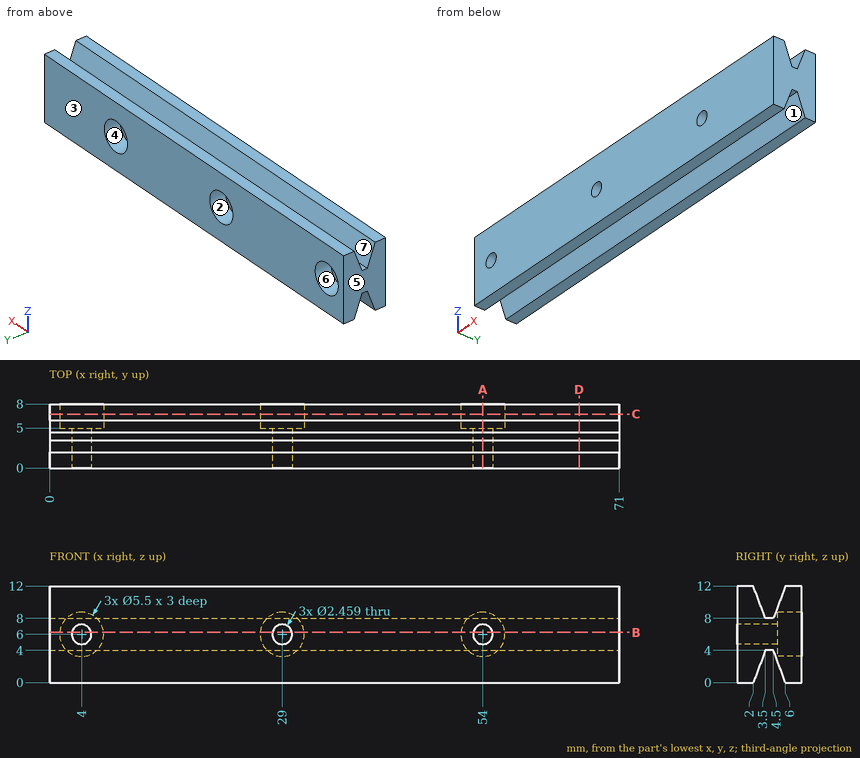
Print and shaded views of the part. All mm, measured from the part's lowest x, y and z. A direction names the side the tool comes from. Round coordinates to 2 decimals unless told otherwise and drop trailing zeros. Write each loop counter-clockwise with the first axis right and the second up, starting at its lowest first coordinate (ties: lowest second). Pieces come first, ordered by that corner, then holes. Notation, with made-up numbers: (2.25, 32) - (45.25, 32) arc R13 ccw to (45.25, 38) - close; hole circle Ø4 at (7, -9). An arc over 180 degrees is marked (long way). One line per question, with ' | ' between items.
1. Mould opens along Z. For the marked faces 4, 5, 6 and 7 say: released by +Z, released by -Z, zero draft, split by the parting line, or undercut.
Results are:
face 4: undercut | face 5: zero draft | face 6: undercut | face 7: released by +Z
2. Band-saw the part on D-D, the plane x = 66. Write the cut outline in (y, z), and give its area (3 significant figures).
Results are:
outline: (0, 0) - (2, 0) - (3.5, 4) - (4.5, 4) - (6, 0) - (8, 0) - (8, 12) - (6, 12) - (4.5, 8) - (3.5, 8) - (2, 12) - (0, 12) - close | area: 76.0 mm^2
3. Drop flat-ended pins along their axis: pin 1 Ø3 at (x, z) = (54, 6) entering from +Y; pin 2 Ø2 at (x, z) = (29, 6) entering from +Y; pin 3 Ø0.8 at (x, y) = (32.5, 4) entering from +Z. Give the stop position or say it passes through.
Results are:
pin 1: y = 5 | pin 2: through | pin 3: z = 8
4. Band-saw the part on A-A, the plane x = 54. Write the cut outline in (y, z).
Results are:
outline: (0, 0) - (2, 0) - (3.5, 4) - (4.5, 4) - (6, 0) - (8, 0) - (8, 3.25) - (5, 3.25) - (5, 4.77) - (0, 4.77) - close; (0, 7.23) - (5, 7.23) - (5, 8.75) - (8, 8.75) - (8, 12) - (6, 12) - (4.5, 8) - (3.5, 8) - (2, 12) - (0, 12) - close
5. Band-saw the part on C-C, the plane y = 6.75. Write the cut outline in (x, z).
Results are:
outline: (0, 0) - (71, 0) - (71, 12) - (0, 12) - close; hole circle Ø5.5 at (4, 6); hole circle Ø5.5 at (29, 6); hole circle Ø5.5 at (54, 6)
6. Band-saw the part on B-B, the plane z = 6.25. Write the cut outline in (x, y), and give its area (3 significant figures).
Results are:
outline: (0, 0) - (2.8, 0) - (2.8, 5) - (1.26, 5) - (1.26, 8) - (0, 8) - close; (5.2, 0) - (27.8, 0) - (27.8, 5) - (26.26, 5) - (26.26, 8) - (6.74, 8) - (6.74, 5) - (5.2, 5) - close; (30.2, 0) - (52.8, 0) - (52.8, 5) - (51.26, 5) - (51.26, 8) - (31.74, 8) - (31.74, 5) - (30.2, 5) - close; (55.2, 0) - (71, 0) - (71, 8) - (56.74, 8) - (56.74, 5) - (55.2, 5) - close | area: 483 mm^2
7. Tool access for the marked faces 1, 2 and 3: list every direction of +Z, -Z, +X, -X, +Y, -Y with a clear straight run to the whole face (end or side of a thin tool).
Results are:
face 1: -Z, +X, -X | face 2: +Y | face 3: +Z, -Z, +X, -X, +Y
8. Drill centre lines: line 1 along X through (y, z) = (7.2, 6); line 2 along X through (y, z) = (1.3, 6); line 3 along Z through (x, y) = (4, 1.5). Where is each one in solid material? Low to high. Write a range as from..to.
Results are:
line 1: 0..1.25, 6.75..26.25, 31.75..51.25, 56.75..71 | line 2: 0..2.77, 5.23..27.77, 30.23..52.77, 55.23..71 | line 3: 0..4.77, 7.23..12
